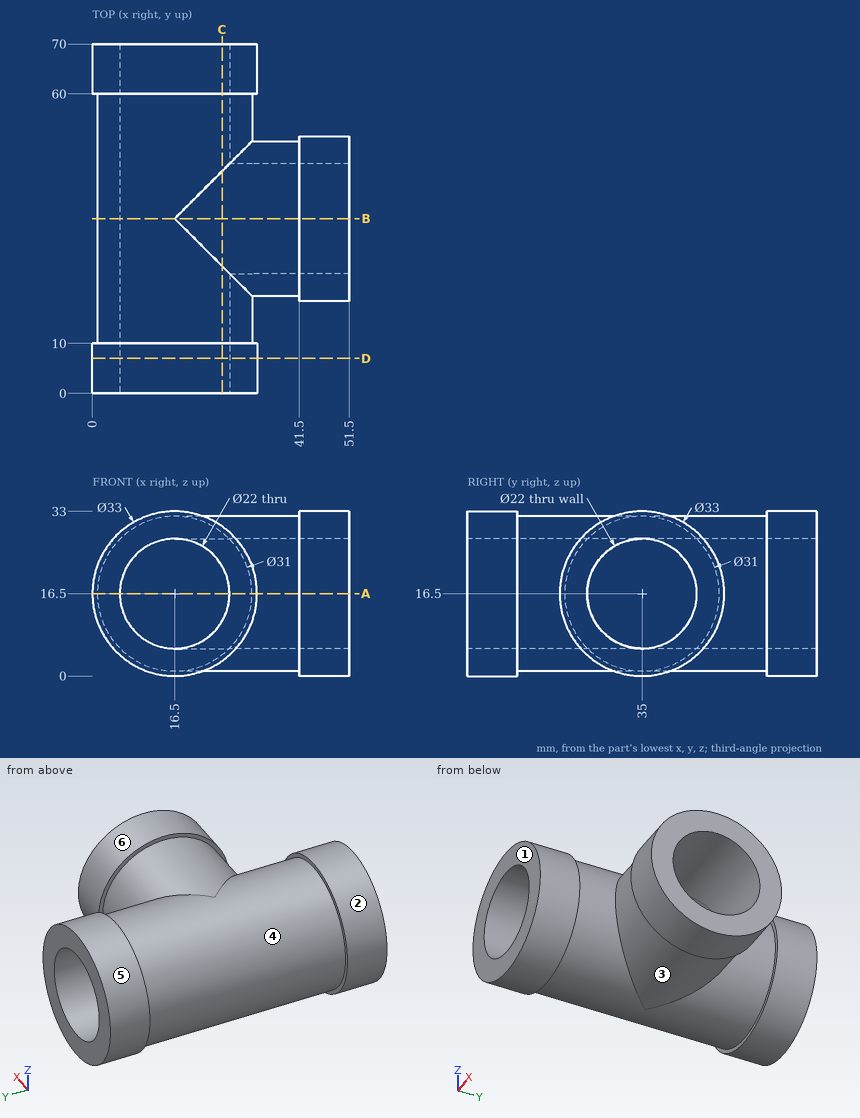
Input: dimensioned drawing with shaded views. Units: mm. Origin: part minimum x, y, z. A direction names the side the tool comes from. Round coordinates to 2 decimals unless told otherwise and drop trailing zeros. Loops run counter-clockwise (first coordinate to the right, second up) from the corner with the lowest first, then second, coordinate; pieces in that order, holes last. Notation, with made-up numbers: M -26,68.5 L 2,68.5 A28 ccw 2,101.5 Z; hole C 8.5,87 d11. An arc over 180 degrees is marked long. Answer in a Markdown table with one row per item. Add a question column.
1. Contact query for flat-ended pins moving along their axis: pin 1 (1 mm diameter, centred on x = 40.5, y = 43, fed in from -Z); pin 2 (17.5 mm diameter, centred on y = 35, z = 16.5, fed in from +X); pin 3 (10 mm diameter, centred on y = 42, z = 10, fed in from -X); pin 4 (6 mm diameter, centred on x = 12, z = 11, fed in from +Y). Output: stop coordinate, or through.
2. Section D-D (y = 7). Output: boundary loops of the cut face in (x, z), and give its area (3 significant figures).
3. Ray query, probe 1 along Z at (x, y) = (20.5, 35); probe 2 along Y at (x, z) = (45.5, 17); probe 3 along Z at (x, y) = (45.75, 35). Return the intervals inside material, ascending.
4. Mould query, pull axis Y, two halves, no side actions, for the marked faces 4, 5 and 6. Classes: released by +Y, released by -Y, zero draft, split by the parting line, or undercut.
5. Section C-C (x = 26). Output: boundary loops of the cut face in (y, z), and give its area (3 significant figures).
6. Section A-A (z = 16.5). Output: boundary loops of the cut face in (x, y), and give its area (4 significant figures).
7. Section B-B (y = 35). Output: boundary loops of the cut face in (x, z).
8. Set-up query: the marked faces 1, 2 and 3. Return all of +Z, -Z, +X, -X, +Y, -Y with unobstructed straight access to the full face (end or side cutting, diameter ignored); none if empty.
Values follow:
| question | item | result |
|---|---|---|
| 1 | pin 1 | z = 2.94 |
| 1 | pin 2 | x = 9.83 |
| 1 | pin 3 | x = 1.07 |
| 1 | pin 4 | through |
| 2 | outline | C 16.5,16.5 d33; hole C 16.5,16.5 d22 |
| 2 | area | 475 mm^2 |
| 3 | probe 1 | 1 to 5.5, 27.5 to 32 |
| 3 | probe 2 | 18.51 to 24.01, 45.99 to 51.49 |
| 3 | probe 3 | 0 to 5.5, 27.5 to 33 |
| 4 | face 4 | undercut |
| 4 | face 5 | zero draft |
| 4 | face 6 | split by the parting line |
| 5 | outline | M 0,3.01 L 10,3.01 L 10,4.25 L 25.5,4.25 A15.5 ccw 44.5,4.25 L 60,4.25 L 60,3.01 L 70,3.01 L 70,10.95 L 44.5,10.95 A11 cw 25.5,10.95 L 0,10.95 Z; M 0,22.05 L 25.5,22.05 A11 cw 44.5,22.05 L 70,22.05 L 70,29.99 L 60,29.99 L 60,28.75 L 44.5,28.75 A15.5 ccw 25.5,28.75 L 10,28.75 L 10,29.99 L 0,29.99 Z |
| 5 | area | 925 mm^2 |
| 6 | outline | M 0,0 L 5.5,0 L 5.5,70 L 0,70 L 0,60 L 1,60 L 1,10 L 0,10 Z; M 27.5,0 L 33,0 L 33,10 L 32,10 L 32,19.5 L 41.5,19.5 L 41.5,18.5 L 51.5,18.5 L 51.5,24 L 27.5,24 Z; M 27.5,46 L 51.5,46 L 51.5,51.5 L 41.5,51.5 L 41.5,50.5 L 32,50.5 L 32,60 L 33,60 L 33,70 L 27.5,70 Z |
| 6 | area | 766.5 mm^2 |
| 7 | outline | M 16.5,1 L 41.5,1 L 41.5,0 L 51.5,0 L 51.5,5.5 L 16.5,5.5 A11 cw 16.5,27.5 L 51.5,27.5 L 51.5,33 L 41.5,33 L 41.5,32 L 16.5,32 A15.5 ccw Z |
| 8 | face 1 | +Z, -Z, +X, -X, -Y |
| 8 | face 2 | -Y |
| 8 | face 3 | none |
